Build history of the part. All positions in model axes, mm. Face numbers are marked on the shaded views. A direction names the side the tool comes from. Give positions to 0.01 mm unless a question says otherwise; leave off trailing zeros. Order: outer loops, then holes, each group sorted by start corner. A loop starts at its lowest first (then second) coordinate and runs counter-clockwise, first axis right, second up. Notation, with made-up numbers: M 24.5,19 L 40.5,19 A19 ccw 40.5,30 Z; hole C 82.5,73 d11. An arc over 180 degrees is marked long. Answer as CSV lines item,"result".
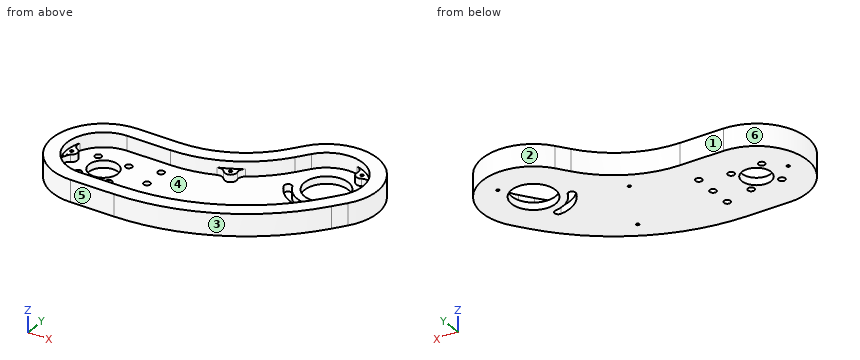
from build123d import *

# Parameters (mm, degrees)
EXTRUDE_1_DEPTH                 = 20
CHAMFER_1_SIZE                  = 10
CUT_EXTRUDE_1_DEPTH             = 15
SKETCH_3_R                      = 15
CUT_EXTRUDE_2_DEPTH             = 20
SKETCH_4_R                      = 2.25
SKETCH_4_R_2                    = 10
CUT_EXTRUDE_3_DEPTH             = 20
SKETCH_5_R                      = 4
EXTRUDE_3_DEPTH                 = 5
FILLET_1_R                      = 5
SKETCH_6_R                      = 1
CUT_EXTRUDE_4_DEPTH             = 10
FILLET_2_R                      = 5
CUT_EXTRUDE_5_REACH             = 22
CUT_EXTRUDE_5_DIRECTION_2_DEPTH = 1.0000001
EXTRUDE_4_DEPTH                 = 13
CUT_EXTRUDE_6_DEPTH             = 5


with BuildPart() as part:
    # 스케치1 → 보스-돌출1 (new body)
    with BuildSketch(Plane.XY):
        with BuildLine():
            Line((0, 35), (30, 35))
            ThreePointArc((30, 35), (61.66442854, 42.571128753), (86.479272356, 63.646743851))
            Line((86.479272356, 63.646743851), (92.386880378, 71.715211331))
            ThreePointArc((92.386880378, 71.715211331), (141.30314463, 79.278219435), (148.866152734, 30.361955182))
            Line((148.866152734, 30.361955182), (142.958544713, 22.293487703))
            ThreePointArc((142.958544713, 22.293487703), (93.328857081, -19.857742494), (30, -35))
            Line((30, -35), (0, -35))
            ThreePointArc((0, -35), (-35, 0), (0, 35))
        make_face()
    extrude(amount=EXTRUDE_1_DEPTH)

    # 모따기1
    chamfer_1_edges = [part.edges().sort_by_distance(p)[0] for p in [
        (141.30314463, 79.278219435, 20),
        (89.433076367, 67.680977591, 20),
        (61.66442854, 42.571128753, 20),
        (15, 35, 20),
        (-35, 0, 20),
        (15, -35, 20),
        (93.328857081, -19.857742494, 20),
        (145.912348723, 26.327721442, 20),
    ]]
    chamfer(chamfer_1_edges, length=CHAMFER_1_SIZE)

    # 스케치2 → 컷-돌출1 (cut)
    with BuildSketch(Plane.XY.offset(20)):
        with BuildLine():
            Line((30, 25), (0, 25))
            ThreePointArc((0, 25), (-25, 0), (0, -25))
            Line((0, -25), (30, -25))
            ThreePointArc((30, -25), (88.805367289, -10.939332316), (134.890077233, 28.201095724))
            Line((134.890077233, 28.201095724), (140.797685254, 36.269563203))
            ThreePointArc((140.797685254, 36.269563203), (135.395536609, 71.209751955), (100.455347857, 65.80760331))
            Line((100.455347857, 65.80760331), (94.547739836, 57.73913583))
            ThreePointArc((94.547739836, 57.73913583), (66.187918332, 33.652718575), (30, 25))
        make_face()
    extrude(amount=-CUT_EXTRUDE_1_DEPTH, mode=Mode.SUBTRACT)

    # 스케치3 → 컷-돌출2 (cut)
    with BuildSketch(Plane.XY.offset(5)):
        with Locations((120.626516556, 51.038583256)):
            Circle(SKETCH_3_R)
    extrude(amount=-CUT_EXTRUDE_2_DEPTH, mode=Mode.SUBTRACT)

    # 스케치4 → 컷-돌출3 (cut)
    with BuildSketch(Plane.XY.offset(5)):
        with Locations((10.606601718, 10.606601718)):
            Circle(SKETCH_4_R)
        with Locations((10.606601718, -10.606601718)):
            Circle(SKETCH_4_R)
        with Locations((-10.606601718, -10.606601718)):
            Circle(SKETCH_4_R)
        with Locations((-10.606601718, 10.606601718)):
            Circle(SKETCH_4_R)
        with Locations((30, 0)):
            Circle(SKETCH_4_R)
        with Locations((30, 15)):
            Circle(SKETCH_4_R)
        with Locations((30, -15)):
            Circle(SKETCH_4_R)
        Circle(SKETCH_4_R_2)
    extrude(amount=-CUT_EXTRUDE_3_DEPTH, mode=Mode.SUBTRACT)

    # 스케치5 → 보스-돌출3 (add)
    with BuildSketch(Plane.XY.offset(5)):
        with Locations((-22, 0)):
            Circle(SKETCH_5_R)
        with Locations((133.623254202, 68.789211711)):
            Circle(SKETCH_5_R)
        with Locations((67.544965269, 30.977195521)):
            Circle(SKETCH_5_R)
        with Locations((87.448320352, -8.263809263)):
            Circle(SKETCH_5_R)
    extrude(amount=EXTRUDE_3_DEPTH)

    # 필렛1
    fillet_1_edges = [part.edges().sort_by_distance(p)[0] for p in [
        (-24.840909091, -2.81588983, 7.5),
        (-24.840909091, 2.81588983, 7.5),
        (133.029560383, 72.744907307, 7.5),
        (137.573543488, 69.417872638, 7.5),
        (68.485091989, 34.865146363, 7.5),
        (63.852594761, 32.515506293, 7.5),
        (91.180070497, -9.703962329, 7.5),
        (86.405731461, -12.125545712, 7.5),
    ]]
    fillet(fillet_1_edges, radius=FILLET_1_R)

    # 스케치6 → 컷-돌출4 (cut)
    with BuildSketch(Plane.XY.offset(10)):
        with Locations((67.544965269, 30.977195521)):
            Circle(SKETCH_6_R)
        with Locations((87.448320352, -8.263809263)):
            Circle(SKETCH_6_R)
        with Locations((-22, 0)):
            Circle(SKETCH_6_R)
        with Locations((133.623254202, 68.789211711)):
            Circle(SKETCH_6_R)
    extrude(amount=-CUT_EXTRUDE_4_DEPTH, mode=Mode.SUBTRACT)

    # 필렛2
    fillet_2_edges = [part.edges().sort_by_distance(p)[0] for p in [
        (141.30314463, 79.278219435, 10),
        (89.433076367, 67.680977591, 10),
        (145.912348723, 26.327721442, 10),
        (61.66442854, 42.571128753, 10),
        (93.328857081, -19.857742494, 10),
        (15, 35, 10),
        (15, -35, 10),
        (-35, 0, 10),
    ]]
    fillet(fillet_2_edges, radius=FILLET_2_R)

    # 스케치7 → 컷-돌출5 (cut, up to next)
    with BuildSketch(Plane(origin=(0, 0, 0), x_dir=(-1, 0, 0), z_dir=(0, 0, -1)), mode=Mode.PRIVATE) as cut_extrude_5_sk1:
        with BuildLine():
            ThreePointArc((-117.92175435, 26.185328713), (-105.857496503, 30.867414558), (-97.750585651, 40.954348766))
            ThreePointArc((-97.750585651, 40.954348766), (-99.029755293, 44.250365305), (-102.325771832, 42.971195664))
            ThreePointArc((-102.325771832, 42.971195664), (-108.811300513, 34.901648297), (-118.462706791, 31.155979621))
            ThreePointArc((-118.462706791, 31.155979621), (-120.677556025, 28.400177947), (-117.92175435, 26.185328713))
        make_face()
    cut_extrude_5_tool1 = extrude(cut_extrude_5_sk1.sketch, amount=-CUT_EXTRUDE_5_REACH, mode=Mode.PRIVATE) & part.part
    add(cut_extrude_5_tool1.solids().sort_by_distance((108.102297, 33.933308, 0))[0], mode=Mode.SUBTRACT)

    # 스케치7 → 컷-돌출5 direction 2 (cut)
    with BuildSketch(Plane(origin=(0, 0, 0), x_dir=(-1, 0, 0), z_dir=(0, 0, -1))):
        with BuildLine():
            ThreePointArc((-117.92175435, 26.185328713), (-105.857496503, 30.867414558), (-97.750585651, 40.954348766))
            ThreePointArc((-97.750585651, 40.954348766), (-99.029755293, 44.250365305), (-102.325771832, 42.971195664))
            ThreePointArc((-102.325771832, 42.971195664), (-108.811300513, 34.901648297), (-118.462706791, 31.155979621))
            ThreePointArc((-118.462706791, 31.155979621), (-120.677556025, 28.400177947), (-117.92175435, 26.185328713))
        make_face()
    extrude(amount=CUT_EXTRUDE_5_DIRECTION_2_DEPTH, mode=Mode.SUBTRACT)

    # 스케치8 → 보스-돌출4 (add)
    with BuildSketch(Plane(origin=(0, 0, 20), x_dir=(-1, 0, 0), z_dir=(0, 0, -1))):
        with BuildLine():
            Line((-30, -35), (0, -35))
            ThreePointArc((0, -35), (35, 0), (0, 35))
            Line((0, 35), (-30, 35))
            ThreePointArc((-30, 35), (-61.66442854, 42.571128753), (-86.479272356, 63.646743851))
            Line((-86.479272356, 63.646743851), (-92.386880378, 71.715211331))
            ThreePointArc((-92.386880378, 71.715211331), (-141.30314463, 79.278219435), (-148.866152734, 30.361955182))
            Line((-148.866152734, 30.361955182), (-142.958544713, 22.293487703))
            ThreePointArc((-142.958544713, 22.293487703), (-93.328857081, -19.857742494), (-30, -35))
        make_face()
        with BuildLine():
            Line((-30, -25), (0, -25))
            ThreePointArc((0, -25), (25, 0), (0, 25))
            Line((0, 25), (-30, 25))
            ThreePointArc((-30, 25), (-66.187918332, 33.652718575), (-94.547739836, 57.73913583))
            Line((-94.547739836, 57.73913583), (-100.455347857, 65.80760331))
            ThreePointArc((-100.455347857, 65.80760331), (-135.395536609, 71.209751955), (-140.797685254, 36.269563203))
            Line((-140.797685254, 36.269563203), (-134.890077233, 28.201095724))
            ThreePointArc((-134.890077233, 28.201095724), (-88.805367289, -10.939332316), (-30, -25))
        make_face(mode=Mode.SUBTRACT)
    extrude(amount=EXTRUDE_4_DEPTH)

    # 스케치9 → 컷-돌출6 (cut)
    with BuildSketch(Plane.XY.offset(20)):
        with BuildLine():
            Line((0, -35), (30, -35))
            ThreePointArc((30, -35), (93.328857081, -19.857742494), (142.958544713, 22.293487703))
            Line((142.958544713, 22.293487703), (148.866152734, 30.361955182))
            ThreePointArc((148.866152734, 30.361955182), (141.30314463, 79.278219435), (92.386880378, 71.715211331))
            Line((92.386880378, 71.715211331), (86.479272356, 63.646743851))
            ThreePointArc((86.479272356, 63.646743851), (61.66442854, 42.571128753), (30, 35))
            Line((30, 35), (0, 35))
            ThreePointArc((0, 35), (-35, 0), (0, -35))
        make_face()
        with BuildLine():
            Line((0, -25), (30, -25))
            ThreePointArc((30, -25), (88.805367289, -10.939332316), (134.890077233, 28.201095724))
            Line((134.890077233, 28.201095724), (140.797685254, 36.269563203))
            ThreePointArc((140.797685254, 36.269563203), (135.395536609, 71.209751955), (100.455347857, 65.80760331))
            Line((100.455347857, 65.80760331), (94.547739836, 57.73913583))
            ThreePointArc((94.547739836, 57.73913583), (66.187918332, 33.652718575), (30, 25))
            Line((30, 25), (0, 25))
            ThreePointArc((0, 25), (-25, 0), (0, -25))
        make_face(mode=Mode.SUBTRACT)
    extrude(amount=-CUT_EXTRUDE_6_DEPTH, mode=Mode.SUBTRACT)


solid = part.part
Item 1: 3-axis set-ups, long thin cutter, end or side, ignore diameter. For the marked faces 1 and 2: which of +Z, -Z, +X, -X, +Y, -Y reach the whole face in a straight line?
Geometry says:
face 1,"+Z, -Z, -X, +Y"
face 2,"+Z, -Z"
Item 2: Probe line 1 along Y through (x, z) = (23, 12.5); line 2 along Y through (x, z) = (109.5, 2); line 3 along X through (y, z) = (2, 1.25). List the from-to ranges inside material, lowest first. Write a range as from..to.
Geometry says:
line 1,"y = -35..-25, 25..35"
line 2,"y = -10.24..28.65, 34.42..40.98, 61.1..84.22"
line 3,"x = -34.94..-9.8, 9.8..28.97, 31.03..124.82"
Item 3: Band-saw the part on C-C (z = 8). State how many separate pieces and enclosed holes the cut face has, and give its area (3 significant figures).
Geometry says:
separate pieces,"1"
enclosed holes,"5"
area,"4,880 mm2"
Item 4: Band-saw the part on A-A (y = 15). Give the cut face in (x, z).
Geometry says:
outline,"M -31.62,0 L 27.75,0 L 27.75,5 L -20,5 L -20,15 L -31.62,15 Z; M 32.25,0 L 137.24,0 L 137.24,15 L 123.81,15 L 123.81,5 L 32.25,5 Z"
Item 5: Pull direction X, two halves, no side cores. Call the marked faces 3, 4, 5 and 6: released by +X, released by -X, zero draft, split by the parting line, or undercut.
Geometry says:
face 3,"released by +X"
face 4,"undercut"
face 5,"zero draft"
face 6,"released by -X"
Item 6: Drop flat-ended pins along their axis: pin 1 (2 mm diameter, centred on x = -15, z = 2.5, fed in from -Y); pin 2 (3.5 mm diameter, centred on x = 30, y = 15, fed in from -Z); pin 3 (1 mm diameter, centred on x = 77.5, z = 9, fed in from -Y); pin 4 (1.5 mm diameter, centred on y = 11.5, z = 8.5, fed in from -X). Give the stop position or say it passes through.
Geometry says:
pin 1,"stops at y = -32.08"
pin 2,"passes through"
pin 3,"stops at y = -26.87"
pin 4,"stops at x = -33.31"
Item 7: Band-saw the part on B-B (x = 25). Give the cut face in (y, z).
Geometry says:
outline,"M -35,0 L 35,0 L 35,15 L 25,15 L 25,5 L -25,5 L -25,15 L -35,15 Z"
Item 8: Band-saw the part on D-D (x = 45). Give the cut face in (y, z), and give its area (3 significant figures).
Geometry says:
outline,"M -34.19,0 L 36.63,0 L 36.63,15 L 26.42,15 L 26.42,5 L -24.13,5 L -24.13,15 L -34.19,15 Z"
area,"557 mm2"
